Input: part model. Units: mm. Frame: model coordinates. Round coordinates to 2 decimals unless told otherwise and drop trailing zeros. Loops run counter-clockwise (first coordinate to the right, second up) from the corner with the lowest first, then second, coordinate; pieces in that order, holes last. Notation, with made-up numbers: M -13,30.5 L 43,30.5 A23 ccw 43,43.5 Z; hole C -10.5,-3 d10. An arc over 180 degrees is marked long. Return JSON: item names as keys, results as strings. Group by question number.
1) Section A-A (y = 0). Output: boundary loops of the cut face in (x, z).
2) Section C-C (z = 1.1). Output: boundary loops of the cut face in (x, y), plus the area to 3 significant figures.
3) Mould query, pull axis Y, two halves, no side actions, for faces 1 (the face through (-77, 1, 3)), 2 (the face through (-9.764, -74.362, 1.479)). Classes: +Y half, -Y half, draft (parallel to the pull), parting line (faces both ways), or undercut.
4) Material intervals for line 1 (Y direction, x = 0, z = 2); line 2 (Y direction, x = 41, z = 1.7); line 3 (X direction, y = 20, z = 0.85), sorted ascending. Write a range as from..to.
Autodesk Inventor part; units mm, degrees
ref_plane "YZ Plane" through (0, 0, 0) normal (1, 0, 0) x (0, 1, 0)
ref_plane "XZ Plane" through (0, 0, 0) normal (0, 1, 0) x (-1, 0, 0)
ref_plane "XY Plane" through (0, 0, 0) normal (0, 0, 1) x (1, 0, 0)
sketch "Sketch1" plane through (0, 0, 0) normal (0, 0, 1) x (1, 0, 0)
  line L0 (-85, -85) -> (85, -85)
  line L1 (85, -85) -> (85, 85)
  line L2 (85, 85) -> (-85, 85)
  line L3 (-85, 85) -> (-85, -85)
  line L4 (-85, -85) -> (85, 85) construction
  line L5 (85, -85) -> (-85, 85) construction
  circle A0 centre (0, 0) radius 75
  dimension "d0" = 170
  dimension "d1" = 170
  dimension "d22" = 150
extrude "Plate1" add sketch "Sketch1" along normal blind 3
equation "\"d1\" = d0"
equation "\"d2\" = Thickness"
equation "\"BendReliefWidth\" = Thickness"
equation "\"BendReliefDepth\" = 0.5 * Thickness"
equation "\"CornerReliefSize\" = 4 * Thickness"
equation "\"MinimumRemnant\" = 2 * Thickness"
equation "\"TransitionRadius\" = BendRadius"
equation "\"JacobiRadiusSize\" = BendRadius"
equation "\"GapSize\" = Thickness"
properties part number "drain bottom plate" material "Stainless Steel"
Returned:
{
 "1": {"outline": "M -85,0 L -75,0 L -75,3 L -85,3 Z; M 75,0 L 85,0 L 85,3 L 75,3 Z"},
 "2": {"outline": "M -85,-85 L 85,-85 L 85,85 L -85,85 Z; hole C 0,0 d150", "area": "11,200 mm^2"},
 "3": {"face 1": "draft", "face 2": "undercut"},
 "4": {"line 1": "y = -85..-75, 75..85", "line 2": "y = -85..-62.8, 62.8..85", "line 3": "x = -85..-72.28, 72.28..85"}
}
